Autodesk Inventor part; units mm, degrees
ref_plane "Work Plane1" through (0, 0, 0) normal (-1, 0, 0) x (0, 0, 1)
ref_plane "YZ Plane" through (0, 0, 0) normal (1, 0, 0) x (0, 1, 0)
ref_plane "XZ Plane" through (0, 0, 0) normal (0, 1, 0) x (-1, 0, 0)
sketch "Sketch1" plane through (0, 0, 0) normal (1, 0, 0) x (0, 1, 0)
  line L0 (0, 0) -> (0, 10.795)
  line L1 (0, 10.795) -> (10.05, 10.795)
  line L2 (10.05, 10.795) -> (10.05, 9.017)
  line L3 (10.05, 9.017) -> (5.8775, 9.017)
  line L4 (5.8775, 9.017) -> (3.81, 1.3008)
  line L5 (4.3488, 0.762) -> (10.05, 0.762)
  line L6 (10.05, 0.762) -> (10.05, 0)
  line L7 (0, 0) -> (10.05, 0) construction
  line L8 (3.81, 1.3008) -> (4.3488, 0.762)
  line L9 (0, 0) -> (0, -10.795)
  line L10 (0, -10.795) -> (10.05, -10.795)
  line L11 (10.05, -10.795) -> (10.05, -9.017)
  line L12 (10.05, -9.017) -> (5.8775, -9.017)
  line L13 (5.8775, -9.017) -> (3.81, -1.3008)
  line L14 (4.3488, -0.762) -> (10.05, -0.762)
  line L15 (10.05, -0.762) -> (10.05, 0)
  line L16 (3.81, -1.3008) -> (4.3488, -0.762)
  dimension "d0" = 10.795
  dimension "d1" = 105
  dimension "d8" = 0.762
  dimension "d33" = 3.81
  dimension "d34" = 10.05
  dimension "d35" = 0.762
  dimension "d36" = 1.778
extrude "Extrusion1" add sketch "Sketch1" along normal mid plane 7.112
sketch "Sketch2" plane through (3.556, 0, 0) normal (1, 0, 0) x (0, 0, -1)
  line L0 (-10.795, 10.05) -> (10.795, 10.05)
  line L1 (10.795, 10.05) -> (10.795, 0)
  line L2 (10.795, 0) -> (-10.795, 0)
  line L3 (-10.795, 0) -> (-10.795, 10.05)
  point P0 (0, 0)
extrude "Extrusion2" add sketch "Sketch2" along normal blind 1.524
ref_plane "Work Plane1" through (0, 0, 0) normal (-1, 0, 0) x (0, 0, 1)
mirror "Mirror1" about plane through (0, 0, 0) normal (-1, 0, 0) of "Extrusion2"
ref_plane "Work Plane2" through (3.556, 5.8775, 0) normal (0, 0, 1) x (1, 0, 0)
sketch "Sketch3" plane through (-3.556, 3.81, -1.3008) normal (0, 0.9659258, 0.258819) x (1, 0, 0)
  circle A0 centre (3.556, 4.4884) radius 2.286
  line L0 (3.556, -2.2426) -> (3.556, 4.4884) construction
  line L1 (7.112, 1.0946) -> (0, 1.0946) construction
  dimension "d14" = 4.572
  dimension "d15" = 6.731
extrude "Extrusion3" cut sketch "Sketch3" against normal blind 1.016
mirror "Mirror2" about plane through (3.556, 5.8775, 0) normal (0, 0, 1) of "Extrusion3"
fillet "Fillet4" radius 3.175 4 edges at (3.556, 7.9638, -9.017) (-3.556, 7.9638, -9.017) (3.556, 7.9638, 9.017) (-3.556, 7.9638, 9.017)
fillet "Fillet5" radius 4.445 4 edges at (5.08, 5.025, 10.795) (5.08, 5.025, -10.795) (-5.08, 5.025, -10.795) (-5.08, 5.025, 10.795)
sketch "Sketch4" plane through (0, 3.9903, 5.8992) normal (0, 0.9659258, -0.258819) x (1, 0, 0)
  line L0 (0, 0.0029) -> (0, -1.1401) construction
  line L1 (0, 0.0029) -> (0, 1.1459) construction
  line L2 (0, 0.0029) -> (0, -1.1079) construction
  circle A0 centre (0, 1.1459) radius 0.8255
  circle A1 centre (0, -1.1401) radius 0.8255
  line L3 (2.1143, 0.0029) -> (2.1143, 2.2658) construction
  point P0 (0, 6.731)
  dimension "d43" = 1.143
  dimension "d44" = 1.651
revolve "Revolution1" cut sketch "Sketch4" angle 90 about axis through (2.1143, 3.9896, 5.8964) along (0, 0.258819, 0.9659258)
mirror "Mirror3" about plane through (3.556, 5.8775, 0) normal (0, 0, 1) of "Revolution1"
sketch "Sketch6" plane through (2.1143, 4.7773, -7.6581) normal (-1, 0, 0) x (0, -1, 0)
  circle A0 centre (2.5341, 0.1105) radius 0.8255
  circle A1 centre (2.5341, 0.1105) radius 0.8255
  circle A2 centre (3.1258, 2.3186) radius 0.8255
  circle A3 centre (3.1258, 2.3186) radius 0.8255
  point P0 (4.7773, 7.6581)
extrude "Extrusion6" cut sketch "Sketch6" against normal up to next
mirror "Mirror10" about plane through (3.556, 5.8775, 0) normal (0, 0, 1) of "Extrusion6"
equation "\"d0\" = 0.5 * Base_Length"
equation "\"d1\" = Sensor_Angle"
equation "\"d33\" = Base_Thickness"
equation "\"d34\" = Mount_Height"
equation "\"d14\" = LED_Base"
equation "\"d15\" = Hole_to_Center"
equation "\"d18\" = Wire_Spacing"
equation "\"Wire_Spacing\" = 1.143"
equation "\"Wire_Diameter\" = 1.651"
equation "\"LED_Base\" = 4.572"
equation "\"Mount_Space\" = 22.75"
equation "\"Mount_Clearance\" = 6.35"
equation "\"Mount_Height\" = 10.05"
equation "\"Base_Length\" = 21.59"
equation "\"Base_Width\" = 10.16"
equation "\"Sensor_Angle\" = 105deg"
equation "\"Base_Thickness\" = 3.81"
equation "\"Hole_to_Center\" = 6.731"
equation "\"Tape_Width\" = 6.35"
properties part number "Line Tracker v4" material "PLA Plastic"
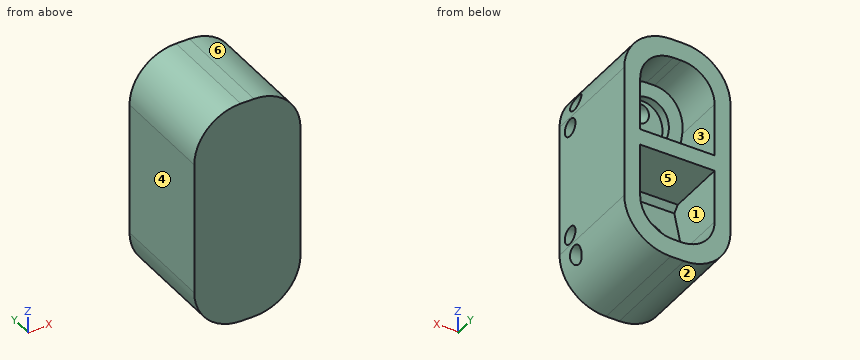
Geometry check sheet. Reference: the model listing, model coordinates, mm. Face numbers are marked on the shaded views. A direction names the side the tool comes from. Give positions to 0.01 mm unless a question says otherwise; leave off trailing zeros. Loops run counter-clockwise (first coordinate to the right, second up) from the corner with the lowest first, then second, coordinate; pieces in that order, holes last.
(1) Section check B-B on x = 4. Record the cut outline in (y, z), then the cut area to 3 significant figures.
From the geometry:
outline: (0, -9.25) - (10.05, -9.25) - (10.05, 9.25) - (0, 9.25) - close; hole circle Ø1.65 at (1.65, -5.34); hole circle Ø1.65 at (1.65, 5.34); hole circle Ø1.65 at (2.24, -7.55); hole circle Ø1.65 at (2.24, 7.55)
area: 177 mm2
(2) Thickness scan on L1, parallel to Z at x = -0.25, y = 7.75 (3 decimals); L2, parallel to X at y = 8.25, z = -5.25; L3, parallel to Z at x = 0, y = 2.25 (3 decimals). Record the ranges inside material, lowest first.
From the geometry:
L1: z = -10.795 to -9.017, -0.762 to 0.762, 9.017 to 10.795
L2: x = -5.08 to -3.56, 3.56 to 5.08
L3: z = -10.795 to -5.797, -4.413 to 4.413, 5.797 to 10.795
(3) Section check C-C on z = -2.25. Record the cut outline in (x, y), then the cut area to 3 significant figures.
From the geometry:
outline: (-5.08, 0) - (5.08, 0) - (5.08, 10.05) - (3.56, 10.05) - (3.56, 4.06) - (-3.56, 4.06) - (-3.56, 10.05) - (-5.08, 10.05) - close
area: 59.5 mm2
(4) Section check D-D on x = -1.75. Record the cut outline in (y, z), then the cut area to 3 significant figures.
From the geometry:
outline: (0, -10.65) - (10.05, -10.65) - (10.05, -8.71) - (5.79, -8.71) - (5.35, -7.06) - (4.37, -7.32) - (3.61, -4.48) - (4.59, -4.22) - (3.81, -1.3) - (4.35, -0.76) - (10.05, -0.76) - (10.05, 0.76) - (4.35, 0.76) - (3.81, 1.3) - (4.59, 4.22) - (3.61, 4.48) - (4.37, 7.32) - (5.35, 7.06) - (5.79, 8.71) - (10.05, 8.71) - (10.05, 10.65) - (0, 10.65) - close
area: 124 mm2
(5) Depth check by flat-ended pin: pin 1 Ø1 at (x, z) = (3, 2.5) entering from +Y; pin 2 Ø4 at (x, y) = (3.5, 7.5) entering from -Z; pin 3 Ø1 at (y, z) = (2.24, -7.55) entering from -X. Enter the tip coordinate at first touch or a pass-through.
From the geometry:
pin 1: stops at y = 4.27
pin 2: stops at z = -10.71
pin 3: stops at x = -5.02
(6) Release check for a two-part mould opening along Z. For the marked faces 3, 4, 5 and 6 record: released by +Z, released by -Z, zero draft, split by the parting line, or undercut.
From the geometry:
face 3: undercut
face 4: zero draft
face 5: undercut
face 6: released by +Z
(7) Section check A-A on y = 6.25. Record the cut outline in (x, z) (3 decimals), then the cut area to 3 significant figures.
From the geometry:
outline: (-5.08, -6.35) arc R4.445 ccw to (-0.635, -10.795) - (0.635, -10.795) arc R4.445 ccw to (5.08, -6.35) - (5.08, 6.35) arc R4.445 ccw to (0.635, 10.795) - (-0.635, 10.795) arc R4.445 ccw to (-5.08, 6.35) - close; hole (-3.556, -5.842) arc R3.175 ccw to (-0.381, -9.017) - (0.381, -9.017) arc R3.175 ccw to (3.556, -5.842) - (3.556, -0.762) - (-3.556, -0.762) - close; hole (-3.556, 0.762) - (3.556, 0.762) - (3.556, 5.842) arc R3.175 ccw to (0.381, 9.017) - (-0.381, 9.017) arc R3.175 ccw to (-3.556, 5.842) - close
area: 93.6 mm2
(8) Set-up check for the marked faces 1 and 2: record each of +Z, -Z, +X, -X, +Y, -Y from which the full face is reachable in a straight line by a thin tool's end or side.
From the geometry:
face 1: +Y
face 2: -Z, -X, +Y, -Y
